Here's the drawing with two shaded views (mm, measured from the low corner). I have some questions. Give positions to 0.01 mm unless a question says otherwise; leave off trailing zeros. Loops run counter-clockwise (first coordinate to the right, second up) from the corner with the lowest first, then second, coordinate; pieces in that order, holes last. Notation, with made-up numbers: M 58.5,16.25 L 77.5,16.25 A18 cw 77.5,25.25 Z; hole C -18.75,34 d1. An arc over 180 degrees is marked long. Use a Markdown table: item, result. Add a question column.
1) Suppose I cut it at D-D on x = 56. List the corners of the cut face in (y, z) for me, and give its area (3 significant figures).
2) If I drill on line 1 along Y through (x, z) = (32, 1.15); line 2 along Y through (x, z) = (32, 4.2); line 3 along Y through (x, z) = (31, 1.9) (1 decimal), over which ranges is the centre line in solid material (lowest first)? Write a range as [from, to].
3) We'd pull the mould along Y, two halves only. Please class the marked faces 1, 2 and 3: +Y half, -Y half, draft (parallel to the pull), parting line (faces both ways), or undercut.
4) Suppose I cut it at A-A on x = 32. List the corners of the cut face in (y, z) for me.
5) Suppose I cut it at B-B on y = 32. List the corners of the cut face in (x, z) for me.
6) Will these pins go through, and if not, where does the flat tip stop? pin 1 Ø12 at (x, y) = (12, 14.5) entering from +Z; pin 2 Ø4 at (x, y) = (44.5, 46) entering from +Z.
7) Suppose I cut it at C-C on z = 4.85. List the corners of the cut face in (x, y) for me, and give its area (3 significant figures).
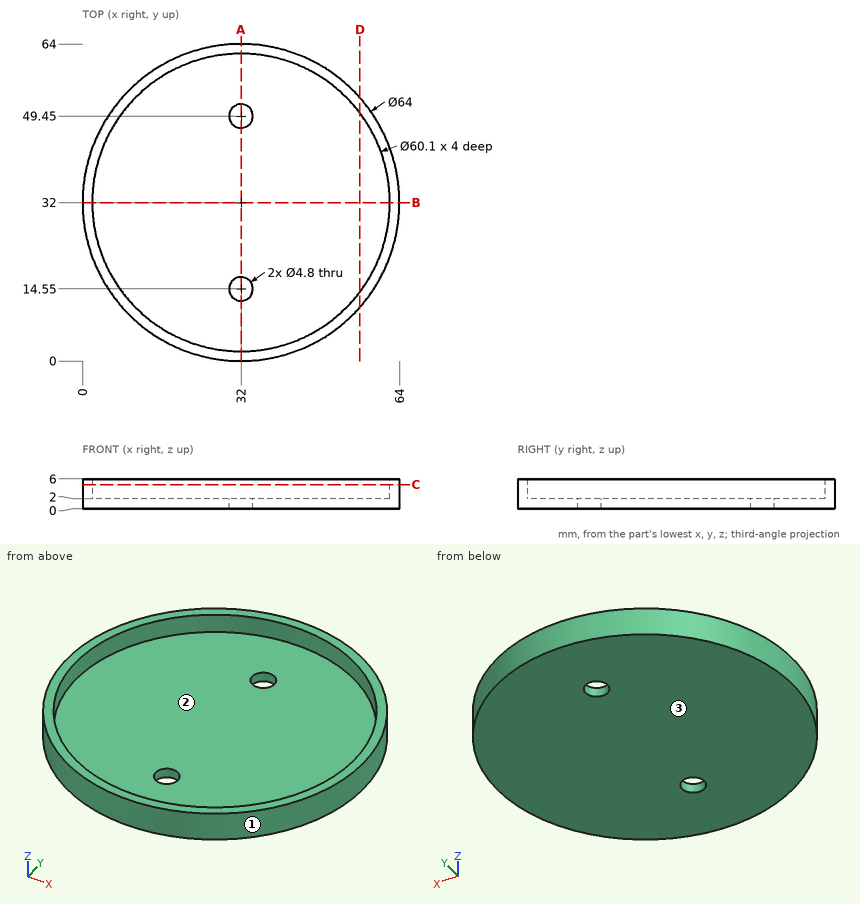
Answer block:
| question | item | result |
|---|---|---|
| 1 | outline | M 10.83,0 L 53.17,0 L 53.17,6 L 50.08,6 L 50.08,2 L 13.92,2 L 13.92,6 L 10.83,6 Z |
| 1 | area | 109 mm^2 |
| 2 | line 1 | y = [0, 12.15], [16.95, 47.05], [51.85, 64] |
| 2 | line 2 | y = [0, 1.95], [62.05, 64] |
| 2 | line 3 | y = [0, 12.4], [16.7, 47.3], [51.6, 64] |
| 3 | face 1 | parting line |
| 3 | face 2 | undercut |
| 3 | face 3 | draft |
| 4 | outline | M 0,0 L 12.15,0 L 12.15,2 L 1.95,2 L 1.95,6 L 0,6 Z; M 16.95,0 L 47.05,0 L 47.05,2 L 16.95,2 Z; M 51.85,0 L 64,0 L 64,6 L 62.05,6 L 62.05,2 L 51.85,2 Z |
| 5 | outline | M 0,0 L 64,0 L 64,6 L 62.05,6 L 62.05,2 L 1.95,2 L 1.95,6 L 0,6 Z |
| 6 | pin 1 | stops at z = 6 |
| 6 | pin 2 | stops at z = 2 |
| 7 | outline | C 32,32 d64; hole C 32,32 d60.1 |
| 7 | area | 380 mm^2 |
